```python
from build123d import *

# Parameters (mm, degrees)
SKETCH_1_W               = 15
SKETCH_1_H               = 5
SKETCH_1_R               = 2.15
SKETCH_1_R_2             = 2.075
EXTRUDE_1_DEPTH          = 8
SKETCH_1_3_R             = 2.075
CUT_EXTRUDE_1_DEPTH      = 2
SKETCH_2_W               = 3
SKETCH_2_H               = 5.4
CUT_EXTRUDE_2_DEPTH      = 3.5
CUT_EXTRUDE_2_DEPTH_BACK = 3.5
EXTRUDE_2_DEPTH          = 2.6
FILLET_1_R               = 2


with BuildPart() as part:
    # 草图1 → 凸台-拉伸1 (new body)
    with BuildSketch(Plane(origin=(0, 0, 0), x_dir=(1, 0, 0), z_dir=(0, 1, 0))):
        Rectangle(SKETCH_1_W, SKETCH_1_H)
        Circle(SKETCH_1_R, mode=Mode.SUBTRACT)
        with Locations((-5, 0)):
            Circle(SKETCH_1_R_2, mode=Mode.SUBTRACT)
        with Locations((5, 0)):
            Circle(SKETCH_1_R_2, mode=Mode.SUBTRACT)
        with Locations((-5, 0)):
            Circle(SKETCH_1_R_2)
        with Locations((5, 0)):
            Circle(SKETCH_1_R_2)
    extrude(amount=EXTRUDE_1_DEPTH)

    # 草图1<3> → 切除-拉伸1 (cut)
    with BuildSketch(Plane(origin=(0, 0, 0), x_dir=(1, 0, 0), z_dir=(0, 1, 0))):
        with Locations((-5, 0)):
            Circle(SKETCH_1_3_R)
        with Locations((5, 0)):
            Circle(SKETCH_1_3_R)
    extrude(amount=CUT_EXTRUDE_1_DEPTH, mode=Mode.SUBTRACT)

    # 草图2 → 切除-拉伸2 (cut, two sides)
    with BuildSketch(Plane.XY) as cut_extrude_2_sk:
        with Locations((-1.5, 5.3)):
            Rectangle(SKETCH_2_W, SKETCH_2_H)
        with Locations((1.5, 5.3)):
            Rectangle(SKETCH_2_W, SKETCH_2_H)
    extrude(amount=CUT_EXTRUDE_2_DEPTH, mode=Mode.SUBTRACT)
    extrude(cut_extrude_2_sk.sketch, amount=-CUT_EXTRUDE_2_DEPTH_BACK, mode=Mode.SUBTRACT)

    # 草图3 → 凸台-拉伸2 (add)
    with BuildSketch(Plane(origin=(0, 0, 0), x_dir=(1, 0, 0), z_dir=(0, 1, 0))):
        Polygon((-1, 4.5), (-3, 2.5), (0, 2.5), (0, 4.5), align=None)
        Polygon((0, 4.5), (0, 2.5), (3, 2.5), (1, 4.5), align=None)
        Polygon((3, -2.5), (0, -2.5), (0, -4.5), (1, -4.5), align=None)
        Polygon((0, -2.5), (-3, -2.5), (-1, -4.5), (0, -4.5), align=None)
    extrude(amount=EXTRUDE_2_DEPTH)

    # 圆角1
    fillet_1_edges = [part.edges().sort_by_distance(p)[0] for p in [
        (7.5, 4, 2.5),
        (-7.5, 4, 2.5),
        (-7.5, 4, -2.5),
        (7.5, 4, -2.5),
    ]]
    fillet(fillet_1_edges, radius=FILLET_1_R)


solid = part.part
```
Read the model definition and answer for the solid it produces. Units are mm, in the model's axes. A direction names the side the tool comes from. Give positions to 0.01 mm unless a question says otherwise; leave off trailing zeros. Write each loop counter-clockwise with the first axis right and the second up, starting at its lowest first coordinate (ties: lowest second). Pieces come first, ordered by that corner, then holes. Notation, with made-up numbers: (-5.5, 21.5) -> (28.5, 21.5) arc R13 cw to (28.5, 33.5) -> close; hole circle Ø10 at (77, 29.25). An arc over 180 degrees is marked (long way). Answer as a JSON object with one key per item and string values.
1) For a pull along Z with two mould halves and no side action, classify faces 4 (the flat face through (4, 4, -2.5)), 5 (the cylindrical face through (-6.65, 0.99, 1.26)), 6 (the flat face through (0, 1, 4.5)), 7 (the flat face through (-5, 8, 0)) as pulls with the +Z half, pulls with the -Z half, needs draft (parallel to the pull), parting line crosses it, or undercut.
Findings below:
{"face 4": "pulls with the -Z half", "face 5": "undercut", "face 6": "pulls with the +Z half", "face 7": "needs draft"}
2) Straight lines are drawn through the part: probe 1 along X at (y, z) = (1.35, 0) (3 decimals); probe 2 along X at (y, z) = (0.5, 1.25); probe 3 along Z at (x, y) = (0, 1.35). For each, find the intervals that lie inside material, in ascending order. Write a range as from..to.
Findings below:
{"probe 1": "x = -7.5..-7.075, -2.925..-2.15, 2.15..2.925, 7.075..7.5", "probe 2": "x = -7.35..-6.66, -3.34..-1.75, 1.75..3.34, 6.66..7.35", "probe 3": "z = -4.5..-2.15, 2.15..4.5"}
3) Section A-A on x = 0 is taken. Write down the section's boundary in (y, z), then the cut area to 3 significant figures.
Findings below:
{"outline": "(0, -4.5) -> (2.6, -4.5) -> (2.6, -2.15) -> (0, -2.15) -> close; (0, 2.15) -> (2.6, 2.15) -> (2.6, 4.5) -> (0, 4.5) -> close", "area": "12.2 mm^2"}
4) Flat-ended cylindrical pins translate along their axes: pin 1 Ø4 at (y, z) = (5.5, 2) entering from -X; pin 2 Ø3 at (x, y) = (-4.5, 3) entering from -Z; pin 3 Ø1.2 at (x, z) = (-5.5, -0.5) entering from -Y; pin 4 Ø2 at (x, y) = (4, 4) entering from +Z. Find the tip coordinate at first contact, or state that the pin passes through.
Findings below:
{"pin 1": "stops at x = -7.5", "pin 2": "stops at z = -2.5", "pin 3": "stops at y = 2", "pin 4": "stops at z = 2.5"}
5) A tool of negligible diameter and unlimited length cuts with its end or side. For faces 1 (the cylindrical face through (3.35, 0.99, 1.26)), 2 (the flat face through (-3, 5, 0)), 3 (the flat face through (-4, 4, -2.5)), from which of +Z, -Z, +X, -X, +Y, -Y can it reach the whole face along a straight path? Write none if from no direction.
Findings below:
{"face 1": "-Y", "face 2": "+Z, -Z, +Y", "face 3": "-Z, -X, +Y, -Y"}
6) Section B-B on y = 6.25 is taken. Write down the section's boundary in (x, z), then the cut area to 3 significant figures.
Findings below:
{"outline": "(-7.5, -0.5) arc R2 ccw to (-5.5, -2.5) -> (-3, -2.5) -> (-3, 2.5) -> (-5.5, 2.5) arc R2 ccw to (-7.5, 0.5) -> close; (3, -2.5) -> (5.5, -2.5) arc R2 ccw to (7.5, -0.5) -> (7.5, 0.5) arc R2 ccw to (5.5, 2.5) -> (3, 2.5) -> close", "area": "41.6 mm^2"}
7) Section C-C on z = 0 is taken. Write down the section's boundary in (x, y) (3 decimals), then the cut area to 3 significant figures.
Findings below:
{"outline": "(-7.5, 0) -> (-7.075, 0) -> (-7.075, 2) -> (-2.925, 2) -> (-2.925, 0) -> (-2.15, 0) -> (-2.15, 2.6) -> (-3, 2.6) -> (-3, 8) -> (-7.5, 8) -> close; (2.15, 0) -> (2.925, 0) -> (2.925, 2) -> (7.075, 2) -> (7.075, 0) -> (7.5, 0) -> (7.5, 8) -> (3, 8) -> (3, 2.6) -> (2.15, 2.6) -> close", "area": "59.8 mm^2"}
8) Section D-D on x = -5 is taken. Write down the section's boundary in (y, z) (3 decimals), then the cut area to 3 significant figures.
Findings below:
{"outline": "(0, -2.5) -> (8, -2.5) -> (8, 2.5) -> (0, 2.5) -> (0, 2.075) -> (2, 2.075) -> (2, -2.075) -> (0, -2.075) -> close", "area": "31.7 mm^2"}
